Part print with two shaded views. Sizes in mm from the minimum x, y, z corner. Round coordinates to 2 decimals unless told otherwise and drop trailing zeros. Write each loop counter-clockwise with the first axis right and the second up, starting at its lowest first coordinate (ties: lowest second). Pieces come first, ordered by that corner, then holes. Notation, with made-up numbers: (-32, -30.75) - (23, -30.75) arc R12 cw to (23, -22.75) - close; hole circle Ø2 at (54, 54). An arc over 180 degrees is marked (long way). Answer as a JSON object with one key per item and string values. Group by question number.
Item 1: Probe line 1 (X direction, y = 3.7, z = 21); line 2 (X direction, y = 0.6, z = 17); line 3 (Y direction, x = 91.5, z = 19). List the from-to ranges inside material, lowest first. Write a range as from..to.
Item 2: Slice it at B-B, the plane y = 1.6. Give the number of separate pieces and of enclosed holes in the cut face, then the cut area to 3 significant figures.
Item 3: Slice it at D-D, the plane x = 3. List the corners of the cut face in (y, z).
Item 4: Flat gauge pins, fed straight in: pin 1 (1 mm diameter, centred on x = 60.5, z = 6, fed in from +Y); pin 2 (1 mm diameter, centred on x = 89, y = 4, fed in from +Z). Where does each tip first touch, or does it go through?
Item 5: Slice it at A-A, the plane x = 89. List the corners of the cut face in (y, z).
Item 6: Slice it at C-C, the plane x = 66.5. List the corners of the cut face in (y, z), then the cut area to 3 significant figures.
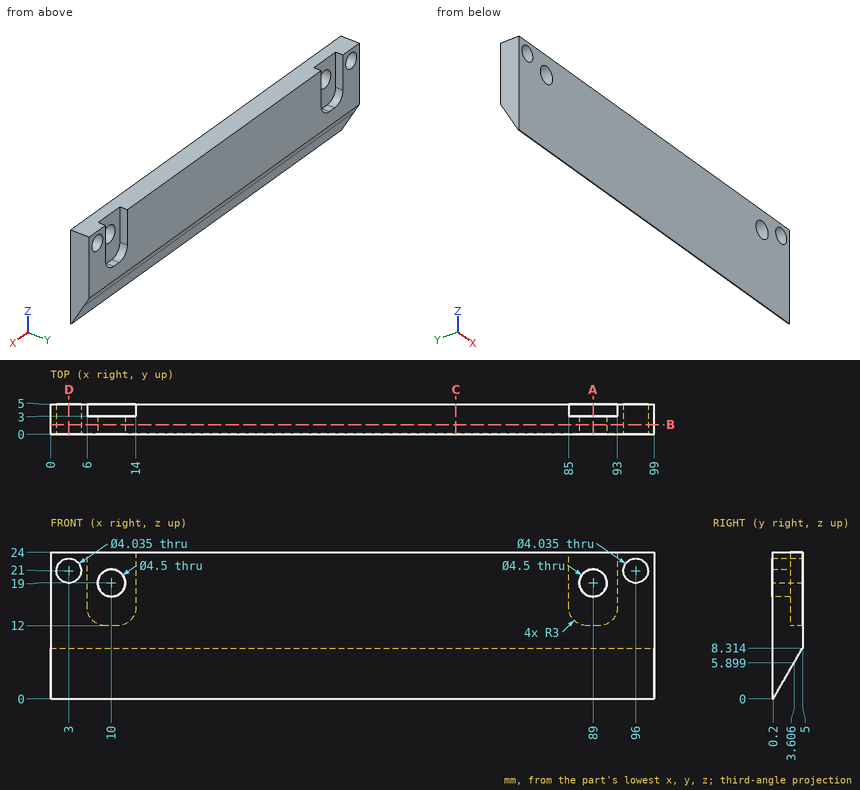
Geometry says:
{
 "1": {"line 1": "x = 0..0.98, 5.02..6, 14..85, 93..93.98, 98.02..99", "line 2": "x = 0..8.97, 11.03..87.97, 90.03..99", "line 3": "y = 0..3"},
 "2": {"separate pieces": "1", "enclosed holes": "4", "area": "2,080 mm^2"},
 "3": {"outline": "(0, 0) - (0.2, 0) - (5, 8.31) - (5, 18.98) - (0, 18.98) - close; (0, 23.02) - (5, 23.02) - (5, 24) - (0, 24) - close"},
 "4": {"pin 1": "stops at y = 3.95", "pin 2": "stops at z = 12"},
 "5": {"outline": "(0, 0) - (0.2, 0) - (5, 8.31) - (5, 12) - (3, 12) - (3, 16.75) - (0, 16.75) - close; (0, 21.25) - (3, 21.25) - (3, 24) - (0, 24) - close"},
 "6": {"outline": "(0, 0) - (0.2, 0) - (5, 8.31) - (5, 24) - (0, 24) - close", "area": "100 mm^2"}
}
